Could you check a few things on this model? Use its own coordinates, in mm. Round coordinates to 2 decimals unless told otherwise and drop trailing zeros. Loops run counter-clockwise (first coordinate to the right, second up) from the corner with the lowest first, then second, coordinate; pieces in that order, holes last. Notation, with made-up numbers: M 62,-38 L 83,-38 A22 cw 83,-26 Z; hole C -8.5,85.5 d5. An arc over 180 degrees is marked long. Return JSON: item names as keys, results as strings. Group by question number.
```python
from build123d import *

# Parameters (mm, degrees)
SKETCH1_R           = 15
SKETCH1_R_2         = 11.5
BOSS_EXTRUDE1_DEPTH = 67.8072
CHAMFER1_SIZE       = 0.25
CHAMFER2_SIZE       = 0.75


with BuildPart() as part:
    # Sketch1 → Boss-Extrude1 (new body)
    with BuildSketch(Plane.XY):
        Circle(SKETCH1_R)
        Circle(SKETCH1_R_2, mode=Mode.SUBTRACT)
    extrude(amount=BOSS_EXTRUDE1_DEPTH)

    # Chamfer1
    chamfer1_edges = [part.edges().sort_by_distance(p)[0] for p in [
        (-15, 0, 0),
        (-15, 0, 67.8072),
    ]]
    chamfer(chamfer1_edges, length=CHAMFER1_SIZE)

    # Chamfer2
    chamfer2_edges = [part.edges().sort_by_distance(p)[0] for p in [
        (-11.5, 0, 0),
        (-11.5, 0, 67.8072),
    ]]
    chamfer(chamfer2_edges, length=CHAMFER2_SIZE)


solid = part.part
```
1. We'd pull the mould along X, two halves only. Please class faces 1 (the face through (-14.985, 0.66, 33.432)), 2 (the face through (-6, 11, 0)), 3 (the face through (-1.5, 11.4, 33.4)): +X half, -X half, draft (parallel to the pull), parting line (faces both ways), or undercut.
2. If we section it at C-C, the plane z = 50.5: Please give me the cut outline in (x, y), then the cut area to 3 significant figures.
3. I'm going to push flat-ended pins straight in: pin 1 Ø4 at (x, z) = (-11.5, 49) entering from -Y; pin 2 Ø1 at (y, z) = (-4.5, 53) entering from +X; pin 3 Ø1 at (x, z) = (-11, 31.5) entering from +Y; pin 4 Ø2 at (x, y) = (-11, -8) entering from -Z. Where does each tip first touch, or does it pass through?
4. I need wall thicknesses on probe 1 along Y at (x, z) = (0, 27.5); probe 2 along X at (y, z) = (5, 34); probe 3 along X at (y, z) = (-2.25, 16). Which ranges of each line are inside material? Lowest first, please.
5. If we section it at A-A, the plane x = 0: Please give me the cut outline in (y, z).
Geometry results:
{
 "1": {"face 1": "parting line", "face 2": "draft", "face 3": "undercut"},
 "2": {"outline": "C 0,0 d30; hole C 0,0 d23", "area": "291 mm^2"},
 "3": {"pin 1": "y = -11.61", "pin 2": "x = 14.46", "pin 3": "y = 10.71", "pin 4": "z = 0"},
 "4": {"probe 1": "-15 to -11.5, 11.5 to 15", "probe 2": "-14.14 to -10.36, 10.36 to 14.14", "probe 3": "-14.83 to -11.28, 11.28 to 14.83"},
 "5": {"outline": "M -15,0.25 L -14.75,0 L -12.25,0 L -11.5,0.75 L -11.5,67.06 L -12.25,67.81 L -14.75,67.81 L -15,67.56 Z; M 11.5,0.75 L 12.25,0 L 14.75,0 L 15,0.25 L 15,67.56 L 14.75,67.81 L 12.25,67.81 L 11.5,67.06 Z"}
}
